Here's the drawing with two shaded views (mm, measured from the low corner). I have some questions. Round coordinates to 2 decimals unless told otherwise and drop trailing zeros. Loops run counter-clockwise (first coordinate to the right, second up) from the corner with the lowest first, then second, coordinate; pieces in that order, holes last.
(1) If I drill on line 1 along Y through (x, z) = (127.6, 1.5); line 2 along X through (y, z) = (48, 1.85); line 3 along Y through (x, z) = (19, 1.4), over which ranges is the centre line in solid material (lowest first)?
(2) I want a section at B-B on x = 95. Write out the boundary of the cut face in (y, z).
(3) I want a section at D-D on y = 65.5. Write out the boundary of the cut face in (x, z).
(4) Will these pins go through, and if not, where does the flat tip stop? pin 1 Ø2.5 at (x, y) = (127.6, 97.6) entering from -Z; pin 2 Ø2 at (y, z) = (2, 1.5) entering from -X; pin 3 Ø2 at (x, z) = (25.5, 2.5) entering from +Y; pin 4 Ø1.2 at (x, z) = (157.5, 2) entering from -Y.
(5) I want a section at A-A on z = 2.75. Write out the boundary of the cut face in (x, y).
(6) I want a section at C-C on y = 97.6. Write out the boundary of the cut face in (x, z).
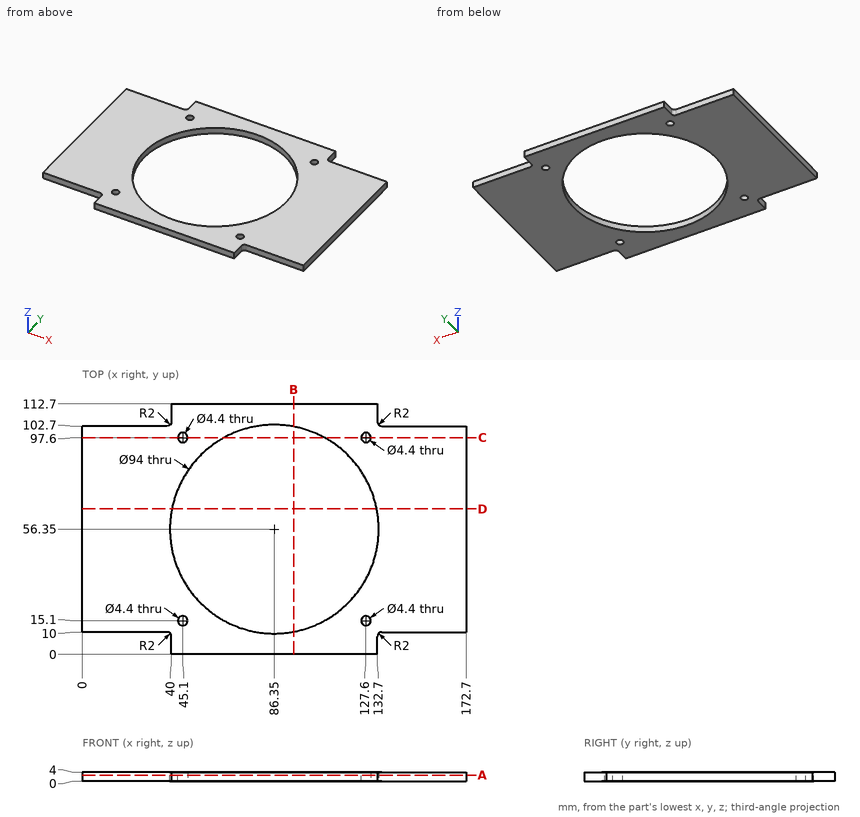
Filled sheet:
1. line 1: y = 0 to 12.9, 17.3 to 33.82, 78.88 to 95.4, 99.8 to 112.7
1. line 2: x = 0 to 40.1, 132.6 to 172.7
1. line 3: y = 10 to 102.7
2. outline: (0, 0) - (10.15, 0) - (10.15, 4) - (0, 4) - close; (102.55, 0) - (112.7, 0) - (112.7, 4) - (102.55, 4) - close
3. outline: (0, 0) - (40.25, 0) - (40.25, 4) - (0, 4) - close; (132.45, 0) - (172.7, 0) - (172.7, 4) - (132.45, 4) - close
4. pin 1: passes through
4. pin 2: stops at x = 40
4. pin 3: stops at y = 102.7
4. pin 4: stops at y = 10
5. outline: (0, 10) - (38, 10) arc R2 cw to (40, 8) - (40, 0) - (132.7, 0) - (132.7, 8) arc R2 cw to (134.7, 10) - (172.7, 10) - (172.7, 102.7) - (134.7, 102.7) arc R2 cw to (132.7, 104.7) - (132.7, 112.7) - (40, 112.7) - (40, 104.7) arc R2 cw to (38, 102.7) - (0, 102.7) - close; hole circle Ø94 at (86.35, 56.35); hole circle Ø4.4 at (45.1, 15.1); hole circle Ø4.4 at (45.1, 97.6); hole circle Ø4.4 at (127.6, 15.1); hole circle Ø4.4 at (127.6, 97.6)
6. outline: (0, 0) - (42.9, 0) - (42.9, 4) - (0, 4) - close; (47.3, 0) - (63.82, 0) - (63.82, 4) - (47.3, 4) - close; (108.88, 0) - (125.4, 0) - (125.4, 4) - (108.88, 4) - close; (129.8, 0) - (172.7, 0) - (172.7, 4) - (129.8, 4) - close
